from build123d import *

# Parameters (mm, degrees)
F1_DEPTH = 1016
F3_DEPTH = 25.4
F5_DEPTH = 25.4
F2_R     = 3.81
F6_DEPTH = 25.4
F7_DEPTH = 25.4


# Not quite as in the source:
# - a feature names something its author has since deleted; it is built from what else it names


with BuildPart() as f1:
    # F0 (on Top) → F1 (new body)
    with BuildSketch(Plane.XY):
        with BuildLine():
            ThreePointArc((12.7, 6.35), (10.8401280605, 10.8401280605), (6.35, 12.7))
            Line((6.35, 12.7), (-6.35, 12.7))
            ThreePointArc((-6.35, 12.7), (-10.8401280605, 10.8401280605), (-12.7, 6.35))
            Line((-12.7, 6.35), (-12.7, -6.35))
            ThreePointArc((-12.7, -6.35), (-10.8401280605, -10.8401280605), (-6.35, -12.7))
            Line((-6.35, -12.7), (6.35, -12.7))
            ThreePointArc((6.35, -12.7), (10.8401280605, -10.8401280605), (12.7, -6.35))
            Line((12.7, -6.35), (12.7, 6.35))
        make_face()
    extrude(amount=F1_DEPTH)

    # F2 (on face) → F3 (cut)
    with BuildSketch(Plane.XZ.offset(12.7)):
        with BuildLine():
            ThreePointArc((3.81, 1003.3), (2.6940768363, 1005.9940768363), (0, 1007.11))
            ThreePointArc((0, 1007.11), (-2.6940768363, 1000.6059231637), (3.81, 1003.3))
        make_face()
    extrude(amount=-F3_DEPTH, mode=Mode.SUBTRACT)

    # F4 (on face) → F5 (cut)
    with BuildSketch(Plane.YZ.offset(12.7)):
        with BuildLine():
            ThreePointArc((3.81, 1003.3), (2.6940768363, 1005.9940768363), (0, 1007.11))
            ThreePointArc((0, 1007.11), (-2.6940768363, 1000.6059231637), (3.81, 1003.3))
        make_face()
    extrude(amount=-F5_DEPTH, mode=Mode.SUBTRACT)

    # F2 (on face) → F6 (cut)
    with BuildSketch(Plane.XZ.offset(12.7)):
        with Locations((0, 749.3)):
            Circle(F2_R)
        with Locations((0, 520.7)):
            Circle(F2_R)
    extrude(amount=-F6_DEPTH, mode=Mode.SUBTRACT)

    # F2 (on face) → F7 (cut)
    with BuildSketch(Plane.XZ.offset(12.7)):
        with Locations((0, 190.5)):
            Circle(F2_R)
    extrude(amount=-F7_DEPTH, mode=Mode.SUBTRACT)


solid = f1.part
Read the model definition and answer for the solid it produces. Units are mm, in the model's axes. Round coordinates to 2 decimals unless told otherwise and drop trailing zeros. Write each loop counter-clockwise with the first axis right and the second up, starting at its lowest first coordinate (ties: lowest second). Pieces come first, ordered by that corner, then holes.
Q1. Find section A-A on z = 822.5. Determine the outline of the cut face in (x, y), and give its area (3 significant figures).
Values:
outline: (-12.7, -6.35) arc R6.35 ccw to (-6.35, -12.7) - (6.35, -12.7) arc R6.35 ccw to (12.7, -6.35) - (12.7, 6.35) arc R6.35 ccw to (6.35, 12.7) - (-6.35, 12.7) arc R6.35 ccw to (-12.7, 6.35) - close
area: 611 mm2
Q2. Straight lines are drawn through the part: line 1 (Z direction, x = 0, y = 1.75); line 2 (Z direction, x = -1, y = 8.75); line 3 (Z direction, x = -5.25, y = 1). For each, find the intervals that lie inside material, in ascending order.
Values:
line 1: z = 0 to 186.69, 194.31 to 516.89, 524.51 to 745.49, 753.11 to 999.49, 1007.11 to 1016
line 2: z = 0 to 186.82, 194.18 to 517.02, 524.38 to 745.62, 752.98 to 999.62, 1006.98 to 1016
line 3: z = 0 to 999.62, 1006.98 to 1016
Q3. Flat-ended cylindrical pins translate along their axes: P1, Ø12, axis at x = 0, z = 190.5, coming from the +Y side; P2, Ø6, axis at y = 0, z = 1003.3, coming from the +X side. Find the tip coordinate at first contact, or state that the pin passes through.
Values:
P1: stops at y = 12.7
P2: passes through
